Read the model definition and answer for the solid it produces. Units are mm, in the model's axes. Face numbers are marked on the shaded views. A direction names the side the tool comes from. Round coordinates to 2 decimals unless told otherwise and drop trailing zeros. Order: outer loops, then holes, each group sorted by start corner. A loop starts at its lowest first (then second) coordinate and runs counter-clockwise, first axis right, second up. Notation, with made-up numbers: (6, 80) -> (36, 80) arc R11 ccw to (36, 96) -> close; hole circle Ø6 at (-21, 85.5). An arc over 180 degrees is marked (long way). Use a Markdown table: item, result. Add a question column.
1. Section A-A, the plane y = -7 is taken. Give the vertices of the cut face in (x, z).
2. Given pin 1 (8.5 mm diameter, centred on y = -9.5, z = 17, fed in from -X); pin 2 (2 mm diameter, centred on x = 16.5, y = -9, fed in from +Z); pin 3 (3 mm diameter, centred on x = 8, y = -5, fed in from -Z); pin 4 (2.5 mm diameter, centred on x = 0, z = 0, fed in from -Y), each flat-ended and moving along its own axis, determine where each tip first touches the part or whether it passes through.
3. Section C-C, the plane x = 0.75 is taken. Give the vertices of the cut face in (y, z), then the cut area to 3 significant figures.
4. For the marked faces 1, 2 and 3, determine the directions among +Z, -Z, +X, -X, +Y, -Y from which every point of the face is accessible in a straight line to the end or side of a thin tool.
5. Consider L1, parallel to X at y = -3.5, z = 9; L2, parallel to Z at x = 0, y = 0.35. Determine where each line is inside the solid, lowest interval first. Write a range as [from, to].
6. Section B-B, the plane z = 0 is taken. Give the vertices of the cut face in (x, y), then the cut area to 3 significant figures.
7. Section D-D, the plane x = 16 is taken. Give the vertices of the cut face in (y, z).
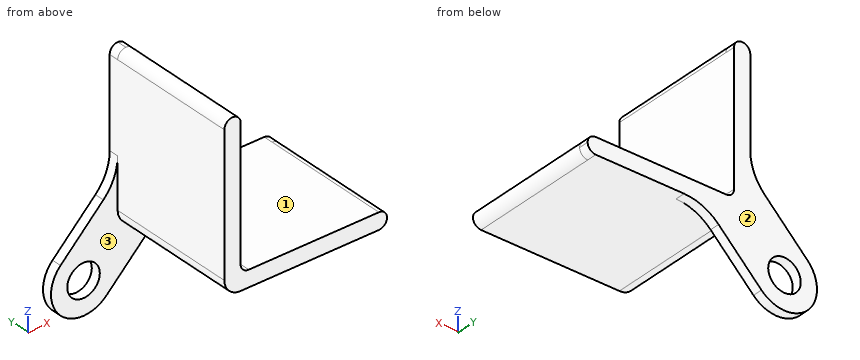
Autodesk Fusion 360 part; units mm, degrees
sketch "Sketch1" plane through (0, 0, 0) normal (0, 1, 0) x (1, 0, 0)
  circle A0 centre (0, 0) radius 2
  line L0 (0, 0) -> (4.2, -4.2) construction
  line L1 (4.2, -4.2) -> (24.2, -4.2)
  line L2 (24.2, -4.2) -> (24.2, -6.2)
  line L3 (24.2, -6.2) -> (4.2, -6.2)
  line L4 (4.2, -6.2) -> (4.2, -4.2)
  line L5 (4.2, -4.2) -> (6.2, -4.2)
  line L6 (6.2, -4.2) -> (6.2, -24.2)
  line L7 (6.2, -24.2) -> (4.2, -24.2)
  line L8 (4.2, -24.2) -> (4.2, -4.2)
  line L9 (4.2, -9.8569) -> (-5.6569, 0)
  line L10 (-5.6569, 0) -> (0, 5.6569)
  line L11 (0, 5.6569) -> (9.8569, -4.2)
  line L12 (0, 0) -> (-2.8284, 2.8284)
  dimension "d1" = 4
  dimension "d2" = 4.2
  dimension "d3" = 4.2
  dimension "d4" = 2
  dimension "d5" = 20
  dimension "d6" = 135
  dimension "d7" = 4
  dimension "d8" = 8
extrude "Extrude1" add sketch "Sketch1" along normal blind 1.2
fillet "Fillet1" radius 1 5 edges at (6.2, 0.6, 6.2) (6.2, 0.6, 24.2) (4.2, 0.6, 24.2) (24.2, 0.6, 6.2) (24.2, 0.6, 4.2)
fillet "Fillet2" radius 4 2 edges at (-5.6569, 0.6, 0) (0, 0.6, -5.6569)
fillet "Fillet3" radius 6 2 edges at (4.2, 0.6, 9.8569) (9.8569, 0.6, 4.2)
sketch "Sketch2" plane through (0, 0, 0) normal (0, -1, 0) x (1, 0, 0)
  arc A0 (-2.8284, 2.8284) -> (2.8284, -2.8284) centre (0, 0) ccw
  line L0 (2.8284, -2.8284) -> (8.0995, 2.4426)
  arc A1 (12.3421, 4.2) -> (8.0995, 2.4426) centre (12.3421, -1.8) ccw
  line L1 (12.3421, 4.2) -> (23.2, 4.2)
  arc A2 (23.2, 4.2) -> (23.2, 6.2) centre (23.2, 5.2) ccw
  line L2 (23.2, 6.2) -> (7.2, 6.2)
  arc A3 (6.2, 7.2) -> (7.2, 6.2) centre (7.2, 7.2) ccw
  line L3 (6.2, 7.2) -> (6.2, 23.2)
  arc A4 (6.2, 23.2) -> (4.2, 23.2) centre (5.2, 23.2) ccw
  line L4 (4.2, 23.2) -> (4.2, 12.3421)
  arc A5 (2.4426, 8.0995) -> (4.2, 12.3421) centre (-1.8, 12.3421) ccw
  line L5 (2.4426, 8.0995) -> (-2.8284, 2.8284)
  circle A6 centre (0, 0) radius 2
  line L6 (4.2, 23.2) -> (4.2, 4.2)
  line L7 (4.2, 4.2) -> (23.2, 4.2)
extrude "Extrude2" add sketch "Sketch2" along normal blind 16 contours L1 A2 L2 A3 L3 A4 L4 L6 L7
fillet "Fillet4" radius 2 1 edges at (4.2, -8, 4.2)
equation "d6 = 180 deg - 45 deg"
Verdict:
| question | item | result |
|---|---|---|
| 1 | outline | (4.2, 6.2) arc R2 ccw to (6.2, 4.2) -> (23.2, 4.2) arc R1 ccw to (23.2, 6.2) -> (7.2, 6.2) arc R1 cw to (6.2, 7.2) -> (6.2, 23.2) arc R1 ccw to (4.2, 23.2) -> close |
| 2 | pin 1 | stops at x = 4.2 |
| 2 | pin 2 | stops at z = 6.2 |
| 2 | pin 3 | stops at z = 4.2 |
| 2 | pin 4 | passes through |
| 3 | outline | (0, -3.93) -> (1.2, -3.93) -> (1.2, -1.85) -> (0, -1.85) -> close; (0, 1.85) -> (1.2, 1.85) -> (1.2, 6.41) -> (0, 6.41) -> close |
| 3 | area | 7.95 mm2 |
| 4 | face 1 | +Z, +X, +Y, -Y |
| 4 | face 2 | +Z, -Z, +X, -X, +Y |
| 4 | face 3 | -Z, -X, -Y |
| 5 | L1 | x = [4.2, 6.2] |
| 5 | L2 | z = [-4, -2], [2, 5.66] |
| 6 | outline | (-4, 0) -> (-2, 0) -> (-2, 1.2) -> (-4, 1.2) -> close; (2, 0) -> (5.66, 0) -> (5.66, 1.2) -> (2, 1.2) -> close |
| 6 | area | 6.79 mm2 |
| 7 | outline | (-16, 4.2) -> (1.2, 4.2) -> (1.2, 6.2) -> (-16, 6.2) -> close |
